Autodesk Inventor part; units mm, degrees
ref_plane "YZ Plane" through (0, 0, 0) normal (1, 0, 0) x (0, 1, 0)
ref_plane "XZ Plane" through (0, 0, 0) normal (0, 1, 0) x (-1, 0, 0)
ref_plane "XY Plane" through (0, 0, 0) normal (0, 0, 1) x (1, 0, 0)
sketch "Sketch1" plane through (0, 0, 0) normal (0, 0, 1) x (1, 0, 0)
  circle A0 centre (0, 0) radius 3.4925
  circle A1 centre (0, 0) radius 2.3495
  line L0 (2.1997, 0) -> (1.0999, -1.905)
  line L1 (1.0999, -1.905) -> (-1.0999, -1.905)
  line L2 (-1.0999, -1.905) -> (-2.1997, 0)
  line L3 (-2.1997, 0) -> (-1.0999, 1.905)
  line L4 (-1.0999, 1.905) -> (1.0999, 1.905)
  line L5 (1.0999, 1.905) -> (2.1997, 0)
  dimension "d0" = 6.985
  dimension "d1" = 4.699
  dimension "d2" = 3.81
extrude "Extrusion1" add sketch "Sketch1" along normal blind 3.81 contours A0 | A1
extrude "Extrusion2" add sketch "Sketch1" against normal blind 5.461 contours A1 | L0 L1 L2 L3 L4 L5
extrude "Extrusion3" add sketch "Sketch1" along normal blind 1.27 contours L0 L1 L2 L3 L4 L5
thread "Thread1"
chamfer "Chamfer1" distance 0.254 angle 45 8 edges at (-3.4925, 0, 3.81) (-3.4925, 0, 0) (-1.6498, 0.9525, 3.81) (-1.6498, -0.9525, 3.81) (0, -1.905, 3.81) (1.6498, -0.9525, 3.81) (1.6498, 0.9525, 3.81) (0, 1.905, 3.81)
properties part number "Gearbox Hex Machine Screw 3" material "Steel"
Could you check a few things on this model? Use its own coordinates, in mm. A direction names the side the tool comes from. Round coordinates to 2 decimals unless told otherwise and drop trailing zeros. Write each loop counter-clockwise with the first axis right and the second up, starting at its lowest first coordinate (ties: lowest second). Pieces come first, ordered by that corner, then holes. Notation, with made-up numbers: M 84.25,17.25 L 109.25,17.25 A25 ccw 109.25,33.25 Z; hole C 40,86.5 d5. An arc over 180 degrees is marked long. Answer in a Markdown table with one row per item. Add a question column.
Q1. If I drill on line 1 (Z direction, x = -3, y = 0.25); line 2 (Z direction, x = 0.5, y = 1); line 3 (Y direction, x = 1.5, z = 2), over which ranges is the centre line in solid material (lowest first)? Write a range as from..to.
Q2. Will these pins go through, and if not, where does the flat tip stop? pin 1 Ø3 at (x, z) = (0, -3.5) entering from -Y; pin 2 Ø1 at (x, z) = (-1.5, 0) entering from +Y.
Q3. Imagine slicing it at C-C (z = 0.75). Please give me the cut outline in (x, y) (1 decimal).
Q4. Imagine slicing it at D-D (z = -4.5). Please give me the cut outline in (x, y).
Q5. If we mould it in two halves opening along X, with no side actions, what happens to faces 3 (the cylindrical face through (-0.31, 2.33, -2.69)), 4 (the flat face through (1.77, 1.002, 3.685)), 5 (the flat face through (2, 2, 0))? For each: +X half, -X half, draft (parallel to the pull), parting line (faces both ways), or undercut.
Q6. Imagine slicing it at A-A (z = 2.5). Please give me the cut outline in (x, y) (1 decimal).
Q7. On a 3-axis mill with a long thin cutter (end or side, diameter ignored), from which of +Z, -Z, +X, -X, +Y, -Y can I reach the whole of each face in a straight line? I mean faces 1 (the flat face through (-1.77, -1.002, 3.685)), 2 (the cylindrical face through (-0.455, -3.463, 1.882)). Say none if no direction works.
Values:
| question | item | result |
|---|---|---|
| 1 | line 1 | 0..3.81 |
| 1 | line 2 | -5.46..1.27 |
| 1 | line 3 | -3.15..-1.21, 1.21..3.15 |
| 2 | pin 1 | y = -2.35 |
| 2 | pin 2 | y = 3.32 |
| 3 | outline | C 0,0 d7 |
| 4 | outline | C 0,0 d4.7 |
| 5 | face 3 | parting line |
| 5 | face 4 | undercut |
| 5 | face 5 | draft |
| 6 | outline | C 0,0 d7; hole M -2.2,0 L -1.1,-1.9 L 1.1,-1.9 L 2.2,0 L 1.1,1.9 L -1.1,1.9 Z |
| 7 | face 1 | +Z |
| 7 | face 2 | +Z, -Z |
